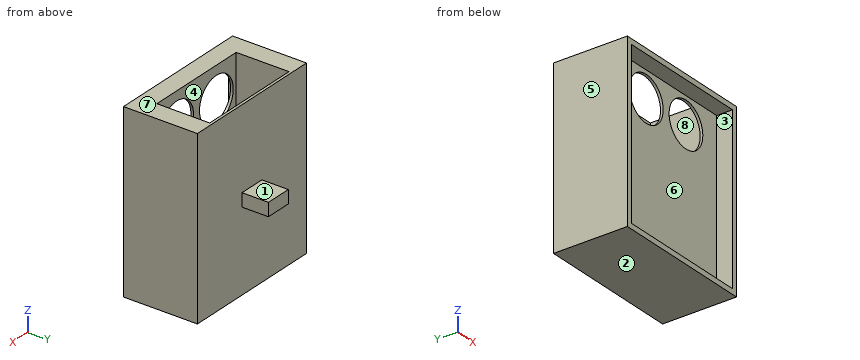
```python
from build123d import *

# Parameters (mm, degrees)
SKETCH1_W           = 69.85
SKETCH1_H           = 6.35
BOSS_EXTRUDE1_DEPTH = 41.91
SHELL1_T            = -2.54
SKETCH2_W           = 69.85
SKETCH2_H           = 83.82
BOSS_EXTRUDE2_DEPTH = 25.4
SKETCH5_W           = 12.7
SKETCH5_H           = 12.7
BOSS_EXTRUDE5_DEPTH = 3.175
SKETCH6_W           = 50.8
SKETCH6_H           = 25.4
CUT_EXTRUDE1_DEPTH  = 30.48
CUT_EXTRUDE2_REACH  = 69.277
SKETCH7_R           = 10.795
SKETCH8_W           = 69.85
SKETCH8_H           = 83.82
SKETCH8_W_2         = 64.77
SKETCH8_H_2         = 78.74
BOSS_EXTRUDE6_DEPTH = 3.81


with BuildPart() as part:
    # Sketch1 → Boss-Extrude1 (new, symmetric)
    with BuildSketch(Plane.XY):
        with Locations((0, 3.175)):
            Rectangle(SKETCH1_W, SKETCH1_H)
    extrude(amount=BOSS_EXTRUDE1_DEPTH, both=True)

    # Shell1
    shell1_openings = [part.faces().sort_by_distance(p)[0] for p in [
        (0, 0, 0),
    ]]
    offset(amount=SHELL1_T, openings=shell1_openings, kind=Kind.INTERSECTION)

    # Sketch2 → Boss-Extrude2 (add)
    with BuildSketch(Plane(origin=(0, 6.35, 0), x_dir=(1, 0, 0), z_dir=(0, 1, 0))):
        Rectangle(SKETCH2_W, SKETCH2_H)
    extrude(amount=BOSS_EXTRUDE2_DEPTH)

    # Sketch5 → Boss-Extrude5 (add, symmetric)
    with BuildSketch(Plane.XY):
        with Locations((0, 38.1)):
            Rectangle(SKETCH5_W, SKETCH5_H)
    extrude(amount=BOSS_EXTRUDE5_DEPTH, both=True)

    # Sketch6 → Cut-Extrude1 (cut)
    with BuildSketch(Plane.XY.offset(41.91)):
        with Locations((0, 17.78)):
            Rectangle(SKETCH6_W, SKETCH6_H)
    extrude(amount=-CUT_EXTRUDE1_DEPTH, mode=Mode.SUBTRACT)

    # Sketch7 → Cut-Extrude2 (cut, up to next)
    with BuildSketch(Plane(origin=(0, 5.08, 0), x_dir=(1, 0, 0), z_dir=(0, 1, 0)), mode=Mode.PRIVATE) as cut_extrude2_sk1:
        with Locations(Location((-12.7, -26.67, 0), (0, 0, 270))):
            Circle(SKETCH7_R)
    cut_extrude2_tool1 = extrude(cut_extrude2_sk1.sketch, amount=-CUT_EXTRUDE2_REACH, mode=Mode.PRIVATE) & part.part
    # Sketch7 → Cut-Extrude2 (cut, up to next)
    with BuildSketch(Plane(origin=(0, 5.08, 0), x_dir=(1, 0, 0), z_dir=(0, 1, 0)), mode=Mode.PRIVATE) as cut_extrude2_sk2:
        with Locations(Location((12.7, -26.67, 0), (0, 0, 270))):
            Circle(SKETCH7_R)
    cut_extrude2_tool2 = extrude(cut_extrude2_sk2.sketch, amount=-CUT_EXTRUDE2_REACH, mode=Mode.PRIVATE) & part.part
    add(cut_extrude2_tool1.solids().sort_by_distance((-12.7, 5.08, 26.67))[0], mode=Mode.SUBTRACT)
    add(cut_extrude2_tool2.solids().sort_by_distance((12.7, 5.08, 26.67))[0], mode=Mode.SUBTRACT)

    # Sketch8 → Boss-Extrude6 (add)
    with BuildSketch(Plane.XZ):
        Rectangle(SKETCH8_W, SKETCH8_H)
        Rectangle(SKETCH8_W_2, SKETCH8_H_2, mode=Mode.SUBTRACT)
    extrude(amount=BOSS_EXTRUDE6_DEPTH)


solid = part.part
```
The model under review builds one solid part; all positions refer to its coordinate system, in mm. Face numbers are marked on the shaded views. A direction names the side the tool comes from. Give positions to 0.01 mm unless a question says otherwise; leave off trailing zeros. Write each loop counter-clockwise with the first axis right and the second up, starting at its lowest first coordinate (ties: lowest second). Pieces come first, ordered by that corner, then holes. Notation, with made-up numbers: (78, 44) -> (100, 44) arc R3 ccw to (100, 49) -> close; hole circle Ø11 at (-6, 34). An arc over 180 degrees is marked (long way). Answer in a Markdown table with one row per item.
1) Add section D-D on z = -13. State the section outline as (x, y) points (3 decimals).
Worked answers:
| item | result |
|---|---|
| outline | (-34.925, -3.81) -> (-32.385, -3.81) -> (-32.385, 3.81) -> (32.385, 3.81) -> (32.385, -3.81) -> (34.925, -3.81) -> (34.925, 31.75) -> (-34.925, 31.75) -> close |
2) Tool access review of the marked faces 1, 2, 3 and 4: name each direction out of +Z, -Z, +X, -X, +Y, -Y from which nothing blocks a thin tool from reaching the whole face with its end or side.
Worked answers:
| item | result |
|---|---|
| face 1 | +Z, +X, -X, +Y |
| face 2 | -Z, +X, -X, +Y, -Y |
| face 3 | -Y |
| face 4 | +Z |
3) Add section B-B on x = 12.7. State the section outline as (y, z) points (3 decimals).
Worked answers:
| item | result |
|---|---|
| outline | (-3.81, -41.91) -> (31.75, -41.91) -> (31.75, 41.91) -> (30.48, 41.91) -> (30.48, 11.43) -> (5.08, 11.43) -> (5.08, 15.875) -> (3.81, 15.875) -> (3.81, -39.37) -> (-3.81, -39.37) -> close; (-3.81, 39.37) -> (3.81, 39.37) -> (3.81, 37.465) -> (5.08, 37.465) -> (5.08, 41.91) -> (-3.81, 41.91) -> close |
4) Add section A-A on z = 26.67. State the section outline as (x, y) points (3 decimals), plus the area to 3 significant figures.
Worked answers:
| item | result |
|---|---|
| outline | (-34.925, -3.81) -> (-32.385, -3.81) -> (-32.385, 3.81) -> (-23.495, 3.81) -> (-23.495, 5.08) -> (-25.4, 5.08) -> (-25.4, 30.48) -> (25.4, 30.48) -> (25.4, 5.08) -> (23.495, 5.08) -> (23.495, 3.81) -> (32.385, 3.81) -> (32.385, -3.81) -> (34.925, -3.81) -> (34.925, 31.75) -> (-34.925, 31.75) -> close; (-1.905, 3.81) -> (1.905, 3.81) -> (1.905, 5.08) -> (-1.905, 5.08) -> close |
| area | 645 mm² |
5) Clearance check with flat-ended pins moving along their axes: P1, Ø4, axis at x = 24.5, z = -7.5, coming from the +Y side; P2, Ø3, axis at x = -3.5, y = 39.5, coming from the -Z side (3 decimals); P3, Ø4, axis at x = -9.5, z = 16.5, coming from the -Y side. State where each tip first meets the part, or that it passes through.
Worked answers:
| item | result |
|---|---|
| P1 | y = 31.75 |
| P2 | z = -3.175 |
| P3 | y = 3.81 |
6) Mouldability with a two-part tool opening along X and no side actions: class the marked faces 5, 6, 7 and 8 as +X half, -X half, draft (parallel to the pull), parting line (faces both ways), or undercut.
Worked answers:
| item | result |
|---|---|
| face 5 | -X half |
| face 6 | undercut |
| face 7 | draft |
| face 8 | undercut |
7) For L1, parallel to X at y = 4, z = 26 (3 decimals); L2, parallel to X at y = 8.5, z = 27.5 (3 decimals); L3, parallel to Z at x = 17.5, y = 3.5, list the stretches that pass through material, from the lowest coordinate up. Write a range as [from, to].
Worked answers:
| item | result |
|---|---|
| L1 | [-34.925, -23.474], [-1.926, 1.926], [23.474, 34.925] |
| L2 | [-34.925, -25.4], [25.4, 34.925] |
| L3 | [-41.91, -39.37], [39.37, 41.91] |
8) Add section C-C on y = 16.5. State the section outline as (x, z) points (3 decimals).
Worked answers:
| item | result |
|---|---|
| outline | (-34.925, -41.91) -> (34.925, -41.91) -> (34.925, 41.91) -> (25.4, 41.91) -> (25.4, 11.43) -> (-25.4, 11.43) -> (-25.4, 41.91) -> (-34.925, 41.91) -> close |
